Can you work these out from the model? Positions are in its coordinate system, mm. Face numbers are marked on the shaded views. A direction names the side the tool comes from. Coordinates: 2 decimals unless noted, no trailing zeros. Write each loop counter-clockwise with the first axis right and the second up, starting at its lowest first coordinate (ties: lowest second). Pieces come first, ordered by that corner, then holes. Notation, with made-up numbers: (15, 67) - (62, 67) arc R19 ccw to (62, 94) - close; hole circle Ø10 at (-37, -14.75). An arc over 180 degrees is marked (long way). Write each question's results on one line, items separated by ' | '. Start each with the question number.
```python
from build123d import *

# Parameters (mm, degrees)
SKETCH_R      = 2.55
PAD_DEPTH     = 6
SKETCH001_R   = 10
SKETCH001_R_2 = 2.466699
PAD001_DEPTH  = 10
FILLET_R      = 0.5


with BuildPart() as part:
    # Sketch → Pad (new body)
    with BuildSketch(Plane.XY):
        Polygon((-6.841601, -3.95), (0, -7.9), (6.841601, -3.95), (6.841601, 3.95), (0, 7.9), (-6.841601, 3.95), align=None)
        Circle(SKETCH_R, mode=Mode.SUBTRACT)
    extrude(amount=PAD_DEPTH)

    # Sketch001 → Pad001 (new body)
    with BuildSketch(Plane(origin=(0, 0, 0), x_dir=(1, 0, 0), z_dir=(0, 0, -1))):
        Circle(SKETCH001_R)
        Circle(SKETCH001_R_2, mode=Mode.SUBTRACT)
    extrude(amount=PAD001_DEPTH)

    # Fillet
    fillet_edges = [part.edges().sort_by_distance(p)[0] for p in [
        (-3.4208, -5.925, 6),
        (3.4208, -5.925, 6),
        (6.841601, 0, 6),
        (3.4208, 5.925, 6),
        (-3.4208, 5.925, 6),
        (-6.841601, 0, 6),
        (-2.55, 0, 6),
    ]]
    fillet(fillet_edges, radius=FILLET_R)


solid = part.part
```
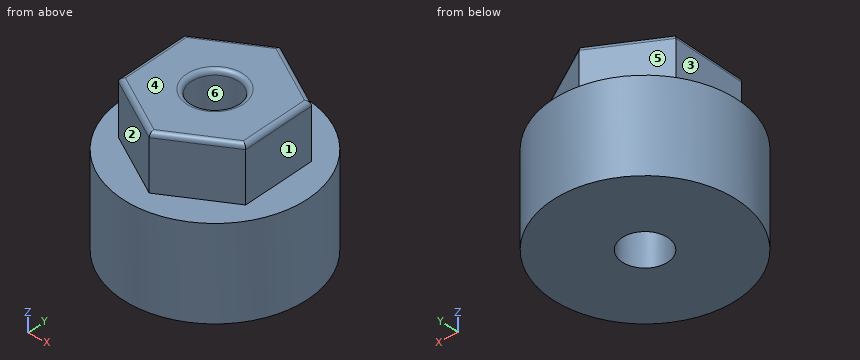
Q1. I'm going to push flat-ended pins straight in: pin 1 Ø6 at (x, z) = (0.5, -6.5) entering from -Y; pin 2 Ø5 at (x, z) = (-4, -6) entering from -Y; pin 3 Ø1 at (y, z) = (7.5, 0) entering from -X; pin 4 Ø6 at (y, z) = (1.5, 3.5) entering from -X. Where does each tip first touch, or does it pass through?
Q2. For the marked faces 1, 2 and 3, which set-ups out of +Z, -Z, +X, -X, +Y, -Y let a thin tool reach every point of the face, with its end or its side?
Q3. If we section it at D-D (z = -1.75): Please give me the cut outline in (x, y).
Q4. If we section it at B-B (z = 4): Please give me the cut outline in (x, y), then the cut area to 3 significant figures.
Q5. I need wall thicknesses on line 1 along Y through (x, z) = (0, -5); line 2 along Z through (x, y) = (-8, 5). Which ranges of each line are inside material? Lowest first, please. Write a range as from..to.
Q6. If we section it at C-C (x = -8.25): Please give me the cut outline in (y, z).
Q7. If we section it at A-A (y = 0): Please give me the cut outline in (x, z), then the cut area to 3 significant figures.
Q8. Thinking about a two-plate mould opening in Y: for the marked faces 4, 5 and 6, which applies, pulls with the +Y half, pulls with the -Y half, needs draft (parallel to the pull), parting line crosses it, or undercut?
Answer list:
1) pin 1: stops at y = -10 | pin 2: stops at y = -9.89 | pin 3: stops at x = -7.14 | pin 4: stops at x = -6.84
2) face 1: +Z, +X, +Y, -Y | face 2: +Z, -X, -Y | face 3: +Z, -X, +Y, -Y
3) outline: circle Ø20 at (0, 0); hole circle Ø4.93 at (0, 0)
4) outline: (-6.84, -3.95) - (0, -7.9) - (6.84, -3.95) - (6.84, 3.95) - (0, 7.9) - (-6.84, 3.95) - close; hole circle Ø5.1 at (0, 0) | area: 142 mm2
5) line 1: y = -10..-2.47, 2.47..10 | line 2: z = -10..0
6) outline: (-5.65, -10) - (5.65, -10) - (5.65, 0) - (-5.65, 0) - close
7) outline: (-10, -10) - (-2.47, -10) - (-2.47, 0) - (-2.55, 0) - (-2.55, 5.5) arc R0.5 ccw to (-3.05, 6) - (-6.34, 6) arc R0.5 ccw to (-6.84, 5.5) - (-6.84, 0) - (-10, 0) - close; (2.47, -10) - (10, -10) - (10, 0) - (6.84, 0) - (6.84, 5.5) arc R0.5 ccw to (6.34, 6) - (3.05, 6) arc R0.5 ccw to (2.55, 5.5) - (2.55, 0) - (2.47, 0) - close | area: 202 mm2
8) face 4: needs draft | face 5: pulls with the +Y half | face 6: undercut
